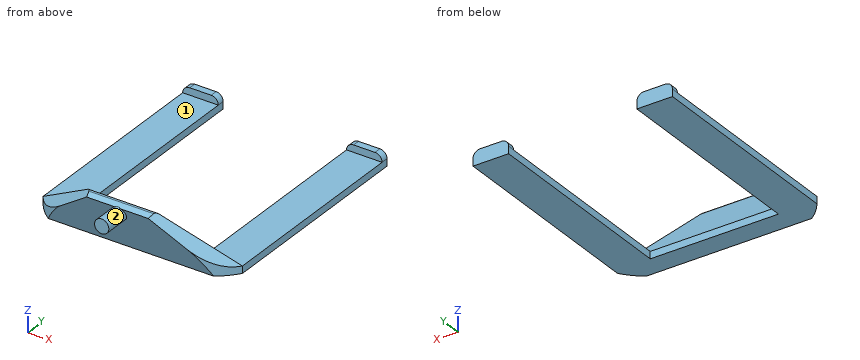
from build123d import *

# Parameters (mm, degrees)
AUFSATZ_LINEAR_AUSTRAGEN1_DEPTH      = 5
SKIZZE2_W                            = 25
SKIZZE2_H                            = 10
AUFSATZ_LINEAR_AUSTRAGEN2_DEPTH      = 5
AUFSATZ_LINEAR_AUSTRAGEN3_DEPTH      = 140
SCHNITT_LINEAR_AUSTRAGEN1_DEPTH      = 20
SKIZZE6_R                            = 5
AUFSATZ_LINEAR_AUSTRAGEN4_DEPTH      = 20
SCHNITT_LINEAR_AUSTRAGEN2_DEPTH      = 5
SCHNITT_LINEAR_AUSTRAGEN3_DEPTH      = 20
SCHNITT_LINEAR_AUSTRAGEN3_DEPTH_BACK = 5
VERRUNDUNG2_R                        = 2


with BuildPart() as part:
    # Skizze1 → Aufsatz-Linear austragen1 (new body)
    with BuildSketch(Plane.XY):
        Polygon((-91.355950116, 49.166666667), (-66.355950116, 49.166666667), (-66.355950116, -90.833333333), (23.644049884, -90.833333333), (23.644049884, 49.166666667), (48.644049884, 49.166666667), (48.644049884, -90.833333333), (48.644049884, -105.833333333), (-91.355950116, -105.833333333), (-91.355950116, -90.833333333), align=None)
    extrude(amount=AUFSATZ_LINEAR_AUSTRAGEN1_DEPTH)

    # Skizze2 → Aufsatz-Linear austragen2 (add)
    with BuildSketch(Plane(origin=(0, 49.166666667, 0), x_dir=(1, 0, 0), z_dir=(0, 1, 0))):
        with Locations((-78.855950116, -5)):
            Rectangle(SKIZZE2_W, SKIZZE2_H)
        with Locations((36.144049884, -5)):
            Rectangle(SKIZZE2_W, SKIZZE2_H)
    extrude(amount=AUFSATZ_LINEAR_AUSTRAGEN2_DEPTH)

    # Skizze4 → Aufsatz-Linear austragen3 (add)
    with BuildSketch(Plane.ZY.offset(91.355950116)):
        Polygon((0, -105.833333333), (33.429341034, -119.769048128), (35.715469601, -114.285025769), (5, -93.839208336), align=None)
    extrude(amount=-AUFSATZ_LINEAR_AUSTRAGEN3_DEPTH)

    # Skizze5 → Schnitt-Linear austragen1 (cut)
    with BuildSketch(Plane(origin=(0, -62.72011839, -41.749779724), x_dir=(1, 0, 0), z_dir=(0, 0.8324398810994642, 0.5541153709789236))):
        Polygon((-91.355950116, -56.159947145), (-41.355950116, -95.491404119), (-91.355950116, -95.491404119), align=None)
        Polygon((48.644049884, -56.159947145), (-1.355950116, -95.491404119), (48.644049884, -95.491404119), align=None)
    extrude(amount=-SCHNITT_LINEAR_AUSTRAGEN1_DEPTH, mode=Mode.SUBTRACT)

    # Skizze6 → Aufsatz-Linear austragen4 (add)
    with BuildSketch(Plane(origin=(0, -115.833333333, 0), x_dir=(1, 0, 0), z_dir=(0, 1, 0))):
        with Locations(Location((-21.355950116, -28.715469601, 0), (0, 0, 180))):
            Circle(SKIZZE6_R)
    extrude(amount=-AUFSATZ_LINEAR_AUSTRAGEN4_DEPTH)

    # Skizze7 → Schnitt-Linear austragen2 (cut)
    with BuildSketch(Plane(origin=(0, 54.166666667, 0), x_dir=(1, 0, 0), z_dir=(0, 1, 0))):
        with BuildLine():
            Line((-91.355950116, -5), (-91.355950116, -10))
            Line((-91.355950116, -10), (-86.355950638, -10))
            ThreePointArc((-86.355950638, -10), (-89.891484175, -8.535533537), (-91.355950116, -5))
        make_face()
        with BuildLine():
            Line((-71.355949595, -10), (-66.355950116, -10))
            Line((-66.355950116, -10), (-66.355950116, -5))
            ThreePointArc((-66.355950116, -5), (-67.820416058, -8.535533537), (-71.355949595, -10))
        make_face()
        with BuildLine():
            Line((23.644049884, -5), (23.644049884, -10))
            Line((23.644049884, -10), (28.644049362, -10))
            ThreePointArc((28.644049362, -10), (25.108515825, -8.535533537), (23.644049884, -5))
        make_face()
        with BuildLine():
            Line((48.644049884, -5), (48.644049884, -10))
            Line((48.644049884, -10), (43.644050405, -10))
            ThreePointArc((43.644050405, -10), (47.179583942, -8.535533537), (48.644049884, -5))
        make_face()
    extrude(amount=-SCHNITT_LINEAR_AUSTRAGEN2_DEPTH, mode=Mode.SUBTRACT)

    # Skizze8 → Schnitt-Linear austragen3 (cut, two sides: drawn at the far end of the back side and taken through both)
    with BuildSketch(Plane.XY.offset(5).offset(-SCHNITT_LINEAR_AUSTRAGEN3_DEPTH_BACK)):
        with BuildLine():
            Line((-91.355950116, -93.839208336), (-91.355950116, -112.568670939))
            Line((-91.355950116, -112.568670939), (-66.355950116, -112.568670939))
            ThreePointArc((-66.355950116, -112.568670939), (-80.35614887, -105.206397991), (-91.355950116, -93.839208336))
        make_face()
        with BuildLine():
            Line((48.644049884, -112.568670939), (23.644049884, -112.568670939))
            ThreePointArc((23.644049884, -112.568670939), (37.644248637, -105.206397991), (48.644049884, -93.839208336))
            Line((48.644049884, -93.839208336), (48.644049884, -112.568670939))
        make_face()
    extrude(amount=SCHNITT_LINEAR_AUSTRAGEN3_DEPTH + SCHNITT_LINEAR_AUSTRAGEN3_DEPTH_BACK, mode=Mode.SUBTRACT)

    # Verrundung2
    verrundung2_edges = [part.edges().sort_by_distance(p)[0] for p in [
        (-21.355950116, -114.285025769, 35.715469601),
    ]]
    fillet(verrundung2_edges, radius=VERRUNDUNG2_R)


solid = part.part
CAD build for the part. Positions are in the model's coordinates, mm. Face numbers are marked on the shaded views. Give positions to 0.01 mm unless a question says otherwise; leave off trailing zeros. Loops run counter-clockwise (first coordinate to the right, second up) from the corner with the lowest first, then second, coordinate; pieces in that order, holes last. Notation, with made-up numbers: M 34,47.25 L 43,47.25 A13 cw 43,57.25 Z; hole C 73.5,74.25 d7. An arc over 180 degrees is marked long. Write each question's results on one line, items separated by ' | '.
Q1. Flat gauge pins, fed straight in: P1, Ø4, axis at x = 32, z = 8.5, coming from the -Y side; P2, Ø1.5, axis at x = -81, z = 8.5, coming from the -Y side; P3, Ø4, axis at x = 1, z = 3, coming from the +Y side; P4, Ø5, axis at x = 32.5, z = 10.5, coming from the +Y side. Where does each tip first touch, or does it go through?
Geometry check:
P1: stops at y = -109.79 | P2: stops at y = -104.83 | P3: stops at y = -90.83 | P4: stops at y = 54.17
Q2. Band-saw the part on D-D on y = -109. Write the cut outline in (x, z).
Geometry check:
outline: M -74.48,7.6 L 31.76,7.6 L 31.76,10.86 L 13.86,27.78 L -56.57,27.78 L -74.48,10.86 Z
Q3. Band-saw the part on C-C on z = 7. Write the cut outline in (x, y).
Geometry check:
outline: M -90.94,49.17 L -66.77,49.17 L -66.77,54.17 L -90.94,54.17 Z; M -88.3,-95.17 L -82.33,-103.65 A50 ccw -74.92,-108.75 L 32.21,-108.75 A50 ccw 39.62,-103.65 L 45.59,-95.17 Z; M 24.06,49.17 L 48.23,49.17 L 48.23,54.17 L 24.06,54.17 Z
Q4. Probe probe 1 along Z at (x, y) = (-81.5, 15); probe 2 along Y at (x, z) = (10, 8.5); probe 3 along Z at (x, y) = (-22, -94). List the from-to ranges inside material, lowest first.
Geometry check:
probe 1: z = 0 to 5 | probe 2: y = -109.38 to -96.17 | probe 3: z = 0 to 5.24
Q5. Mould opens along Y. For the marked faces 1 and 2 say: pulls with the +Y half, pulls with the -Y half, needs draft (parallel to the pull), parting line crosses it, or undercut.
Geometry check:
face 1: undercut | face 2: needs draft
Q6. Band-saw the part on B-B on x = -38. Write the cut outline in (y, z), and give its area (3 significant figures).
Geometry check:
outline: M -119.77,33.43 L -105.83,0 L -90.83,0 L -90.83,5 L -93.84,5 L -113.37,34.34 A2 ccw -115.81,35.08 Z | area: 387 mm²
Q7. Band-saw the part on A-A on y = -25. Write the cut outline in (x, z).
Geometry check:
outline: M -91.36,0 L -66.36,0 L -66.36,5 L -91.36,5 Z; M 23.64,0 L 48.64,0 L 48.64,5 L 23.64,5 Z
